Read the model definition and answer for the solid it produces. Units are mm, in the model's axes. Face numbers are marked on the shaded views. A direction names the side the tool comes from. Give positions to 0.01 mm unless a question says otherwise; leave off trailing zeros. Loops run counter-clockwise (first coordinate to the right, second up) from the corner with the lowest first, then second, coordinate; pieces in that order, holes last. Notation, with made-up numbers: (-14, 21.5) - (0, 21.5) arc R9 ccw to (0, 29.5) - close; hole circle Ø5 at (13.5, 9). An arc over 180 degrees is marked (long way). Use a Markdown table: item, result. Add a question column.
Item 1: Each of these flat-tipped pins is pushed along its axis until it touches: P1, Ø20.5, axis at x = 0, z = 0, coming from the -Y side; P2, Ø2, axis at x = 19, y = 25, coming from the +Z side; P3, Ø12, axis at y = 21, z = 4.5, coming from the -X side; P4, Ø3, axis at x = 8, z = -7, coming from the +Y side. Where does it stop, or does it pass through?
Item 2: Which of the six approach directions +Z, -Z, +X, -X, +Y, -Y give full straight-line access (tool end or side, diameter ignored) to the marked faces 4, 5 and 6?
Item 3: For a pull along Z with two mould halves and no side action, classify the marked faces 1, 2 and 3 as +Z half, -Z half, draft (parallel to the pull), parting line (faces both ways), or undercut.
Item 4: A cutting plane is placed at B-B (y = 37). Determine the outline of the cut face in (x, z), plus the area to 3 significant figures.
Item 5: A cutting plane is placed at A-A (y = 14). Determine the outline of the cut face in (x, z), plus the area to 3 significant figures.
Item 6: A cutting plane is placed at C-C (z = -2.5). Give the number of separate pieces and of enclosed holes in the cut face, plus the area to 3 significant figures.
Item 7: Consider probe 1 along X at (y, z) = (-7, 0); probe 2 along Y at (x, z) = (-18, 7.5); probe 3 along Y at (x, z) = (-3, 18). Determine where each line is inside the solid, lowest interval first. Write a range as [from, to].
from build123d import *

# Parameters (mm, degrees)
BOSS_EXTRUDE1_DEPTH = 26


with BuildPart() as part:
    # Sketch1 → Revolve-Thin3 (revolve)
    with BuildSketch(Plane.XY, mode=Mode.PRIVATE) as revolve_thin3_sk:
        Polygon((-20, 13.228756555), (-18, 13.228756555), (-9, 0), (-9, -10), (-11, -10), (-11, -0.615831877), (-19.058300524, 11.228756555), (-20, 11.228756555), align=None)
    revolve(revolve_thin3_sk.sketch.rotate(Axis((0, 0, 0), (0, 1, 0)), 270), axis=Axis((0, 0, 0), (0, 1, 0)))



with BuildPart() as body_2:
    # Sketch5 → Revolve-Thin5 (revolve)
    with BuildSketch(Plane.XY, mode=Mode.PRIVATE) as revolve_thin5_sk:
        Polygon((1.428130018, 21.872546541), (18, 38.444416522), (20, 38.444416522), (20, 40.444416522), (17.171572875, 40.444416522), (0.013916456, 23.286760103), align=None)
    revolve(revolve_thin5_sk.sketch.rotate(Axis((0, 0, 0), (0, 1, 0)), 270), axis=Axis((0, 0, 0), (0, 1, 0)))


with BuildPart() as part_1:
    add(part.part)

    add(body_2.part)  # Boss-Extrude1 merges body 2
    # Sketch7 → Boss-Extrude1 (add)
    with BuildSketch(Plane.XZ.offset(-38.444416522)):
        Polygon((-18.203416664, 8.284661837), (-16.298741538, 7.638784214), (-17.583300095, 3.850656798), (-19.487975221, 4.496534421), align=None)
        Polygon((17.046573369, -5.780513503), (16.231562144, -7.780513503), (18.0866902, -8.536488599), (19.639442906, -3.780513503), (17.598514643, -3.780513503), align=None)
    extrude(amount=BOSS_EXTRUDE1_DEPTH)


solid = part_1.part
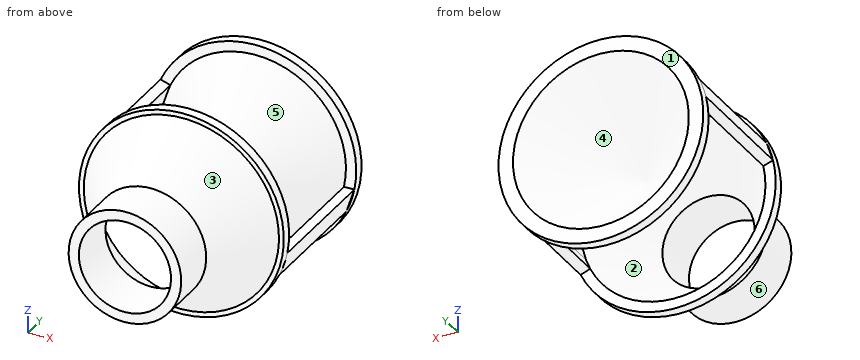
Geometry says:
| question | item | result |
|---|---|---|
| 1 | P1 | y = -10 |
| 1 | P2 | z = -3.78 |
| 1 | P3 | x = -19.49 |
| 1 | P4 | y = 35.4 |
| 2 | face 4 | +Y |
| 2 | face 5 | none |
| 2 | face 6 | -Y |
| 3 | face 1 | draft |
| 3 | face 2 | undercut |
| 3 | face 3 | parting line |
| 4 | outline | (-19.49, 4.5) - (-17.58, 3.85) - (-16.3, 7.64) - (-18.2, 8.28) - close; circle Ø33.11 at (0, 0); (16.23, -7.78) - (18.09, -8.54) - (19.64, -3.78) - (17.6, -3.78) - (17.05, -5.78) - close; hole circle Ø27.45 at (0, 0) |
| 4 | area | 286 mm² |
| 5 | outline | (-19.49, 4.5) - (-17.58, 3.85) - (-16.3, 7.64) - (-18.2, 8.28) - close; (16.23, -7.78) - (18.09, -8.54) - (19.64, -3.78) - (17.6, -3.78) - (17.05, -5.78) - close |
| 5 | area | 16.9 mm² |
| 6 | separate pieces | 3 |
| 6 | enclosed holes | 0 |
| 6 | area | 216 mm² |
| 7 | probe 1 | [-11, -9], [9, 11] |
| 7 | probe 2 | [11.23, 40.44] |
| 7 | probe 3 | [10.04, 13.23], [38.44, 40.44] |
